```python
from build123d import *

# Parameters (mm, degrees)
F0_R     = 3
F1_DEPTH = 3


with BuildPart() as f1:
    # F0 (on Front) → F1 (new body)
    with BuildSketch(Plane.XZ):
        with BuildLine():
            Line((7.75, -6.655555), (7.75, 7.75))
            Line((7.75, 7.75), (7.693235, 7.75))
            ThreePointArc((7.693235, 7.75), (0, 15.443235), (-7.693235, 7.75))
            Line((-7.693235, 7.75), (-7.75, 7.75))
            Line((-7.75, 7.75), (-7.75, -6.655555))
            ThreePointArc((-7.75, -6.655555), (0, -15.576897), (7.75, -6.655555))
        make_face()
        Circle(F0_R, mode=Mode.SUBTRACT)
    extrude(amount=F1_DEPTH)


solid = f1.part
```
Design review of the part built by this model. Coordinates are the model's own, in mm. A direction names the side the tool comes from. Round coordinates to 2 decimals unless told otherwise and drop trailing zeros. Order: outer loops, then holes, each group sorted by start corner. A loop starts at its lowest first (then second) coordinate and runs counter-clockwise, first axis right, second up. Notation, with made-up numbers: M -29,-18 L -17,-18 A28 ccw -17,7 Z; hole C -19,17 d10. An arc over 180 degrees is marked long. Put each result on its own line as item: value.
Q1. Machinability: for faces 4 (the face through (7.75, -1, 0)), 5 (the face through (-7.75, -1, 1)), 6 (the face through (-0.1, -3, -3.3)), which of the approach directions +Z, -Z, +X, -X, +Y, -Y give a long, thin tool a straight path to every point of the face, cutting with its end or side? Answer none if there is none.
Reported:
face 4: +Z, +X, +Y, -Y
face 5: +Z, -X, +Y, -Y
face 6: +Z, -Z, +X, -X, -Y
Q2. To check wall thickness, follow line 1 (Z direction, x = 0, y = -1.3); line 2 (X direction, y = -2, z = -6.5); line 3 (Z direction, x = -0.75, y = -2.6). State the ranges of each line that lie inside material, in increasing order.
Reported:
line 1: -15.58 to -3, 3 to 15.44
line 2: -7.75 to 7.75
line 3: -15.54 to -2.9, 2.9 to 15.41
Q3. Consider section C-C (y = -0.6). State the section outline as (x, z) points, and give its area (3 significant figures).
Reported:
outline: M -7.75,-6.66 A7.83 ccw long 7.75,-6.66 L 7.75,7.75 L 7.69,7.75 A7.69 ccw -7.69,7.75 L -7.75,7.75 Z; hole C 0,0 d6
area: 401 mm²
Q4. Insertion check: pin 1 Ø0.9 at (y, z) = (-2, -1) entering from -X; pin 2 Ø1.5 at (y, z) = (-2, 3.5) entering from +X. Each pin has a flat end and moves straight along its axis. Give the tip position at first contact, or say it passes through.
Reported:
pin 1: x = -7.75
pin 2: x = 7.75
Q5. Draft analysis for pull direction Z (two halves, no side actions). For faces 1 (the face through (-0.1, 0, -3.3)), 2 (the face through (0.17, -1.48, 15.44)), 3 (the face through (-3, -1, 0)), state which applies: released by +Z, released by -Z, zero draft, split by the parting line, or undercut.
Reported:
face 1: zero draft
face 2: released by +Z
face 3: undercut
Q6. Consider section A-A (z = 0). State the section outline as (x, y) points, and give its area (3 significant figures).
Reported:
outline: M -7.75,-3 L -3,-3 L -3,0 L -7.75,0 Z; M 3,-3 L 7.75,-3 L 7.75,0 L 3,0 Z
area: 28.5 mm²
Q7. Consider section D-D (x = 5.5). State the section outline as (y, z) points, and give its area (3 significant figures).
Reported:
outline: M -3,-13.32 L 0,-13.32 L 0,13.13 L -3,13.13 Z
area: 79.3 mm²
Q8. Consider section B-B (x = 0). State the section outline as (y, z) points.
Reported:
outline: M -3,-15.58 L 0,-15.58 L 0,-3 L -3,-3 Z; M -3,3 L 0,3 L 0,15.44 L -3,15.44 Z
